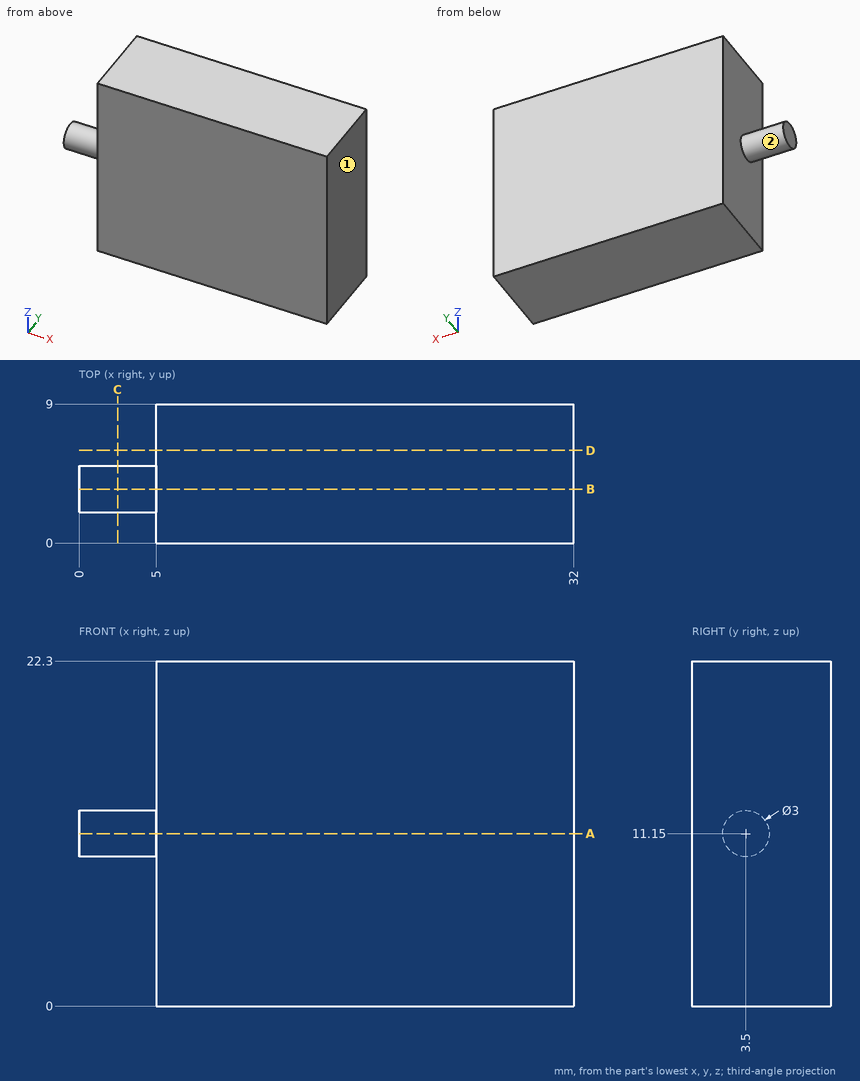
Study the drawing (mm; zero at the part's minimum x, y, z) and answer. A direction names the side the tool comes from. Give positions to 0.01 mm unless a question says otherwise; leave off trailing zeros. Write each loop counter-clockwise with the first axis right and the second up, starting at its lowest first coordinate (ties: lowest second). Pieces come first, ordered by that corner, then holes. Notation, with made-up numbers: (82, 29) -> (120, 29) arc R28 ccw to (120, 61) -> close; hole circle Ø3 at (55.5, 78.25). An arc over 180 degrees is marked (long way). Answer as a JSON object with one key per item and string values. Group by question number.
1) Find section A-A (z = 11.15). Write down the section's boundary in (x, y), and give its area (3 significant figures).
2) Consider L1, parallel to X at y = 4.5, z = 1.75. Determine where the line is inside the solid, lowest interval first. Write a range as from..to.
3) Find section C-C (x = 2.5). Write down the section's boundary in (y, z), and give its area (3 significant figures).
4) This flat-tipped pin is pushed along its axis until it touches: P1, Ø1, axis at y = 1.5, z = 5.5, coming from the -X side. Where does it stop, or does it pass through?
5) Find section B-B (y = 3.5). Write down the section's boundary in (x, z), and give its area (3 significant figures).
6) Find section D-D (y = 6). Write down the section's boundary in (x, z), and give its area (3 significant figures).
7) A tool of negligible diameter and unlimited length cuts with its end or side. For the marked faces 1 and 2, from which of +Z, -Z, +X, -X, +Y, -Y can it reach the whole face along a straight path? Write none if from no direction.
Values follow:
{
 "1": {"outline": "(0, 2) -> (5, 2) -> (5, 0) -> (32, 0) -> (32, 9) -> (5, 9) -> (5, 5) -> (0, 5) -> close", "area": "258 mm2"},
 "2": {"L1": "x = 5..32"},
 "3": {"outline": "circle Ø3 at (3.5, 11.15)", "area": "7.07 mm2"},
 "4": {"P1": "stops at x = 5"},
 "5": {"outline": "(0, 9.65) -> (5, 9.65) -> (5, 0) -> (32, 0) -> (32, 22.3) -> (5, 22.3) -> (5, 12.65) -> (0, 12.65) -> close", "area": "617 mm2"},
 "6": {"outline": "(5, 0) -> (32, 0) -> (32, 22.3) -> (5, 22.3) -> close", "area": "602 mm2"},
 "7": {"face 1": "+Z, -Z, +X, +Y, -Y", "face 2": "-X"}
}
